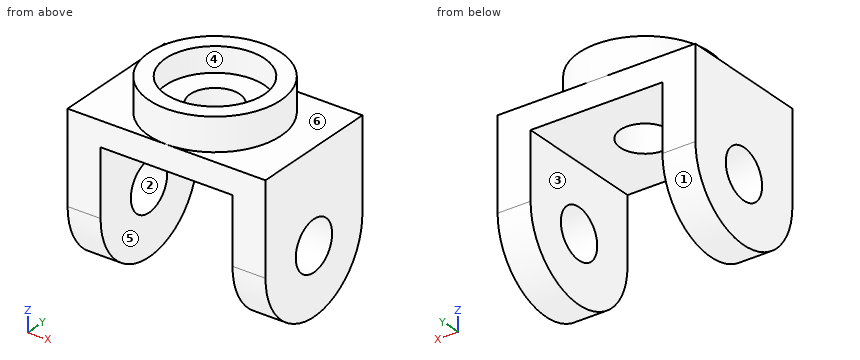
from build123d import *

# Parameters (mm, degrees)
SKETCH_W        = 120
SKETCH_H        = 80
PAD_DEPTH       = 15
SKETCH001_R     = 40
PAD001_DEPTH    = 20
SKETCH002_R     = 30
POCKET_DEPTH    = 15
SKETCH003_R     = 15
POCKET001_DEPTH = 20.001
SKETCH004_R     = 15
PAD002_DEPTH    = 120
SKETCH005_W     = 80
SKETCH005_H     = 96.232483
POCKET002_DEPTH = 80.0010000001


with BuildPart() as part:
    # Sketch → Pad (new body)
    with BuildSketch(Plane.XY):
        Rectangle(SKETCH_W, SKETCH_H)
    extrude(amount=-PAD_DEPTH)

    # Sketch001 → Pad001 (new body)
    with BuildSketch(Plane.XY):
        Circle(SKETCH001_R)
    extrude(amount=PAD001_DEPTH)

    # Sketch002 → Pocket (cut)
    with BuildSketch(Plane.XY.offset(20)):
        Circle(SKETCH002_R)
    extrude(amount=-POCKET_DEPTH, mode=Mode.SUBTRACT)

    # Sketch003 → Pocket001 (cut, through all)
    with BuildSketch(Plane.XY.offset(5)):
        Circle(SKETCH003_R)
    extrude(amount=-POCKET001_DEPTH, mode=Mode.SUBTRACT)

    # Sketch004 → Pad002 (new body)
    with BuildSketch(Plane.YZ.offset(60)):
        with BuildLine():
            ThreePointArc((-40, -55), (3.45478e-05, -95), (39.9999999999, -54.9999309045))
            Line((39.9999999999, -15), (39.9999999999, -54.9999309045))
            Line((-40, -15), (39.9999999999, -15))
            Line((-40, -55), (-40, -15))
        make_face()
        with Locations((0, -55)):
            Circle(SKETCH004_R, mode=Mode.SUBTRACT)
    extrude(amount=-PAD002_DEPTH)

    # Sketch005 → Pocket002 (cut, through all)
    with BuildSketch(Plane.XZ.offset(40)):
        with Locations((0, -63.1162415)):
            Rectangle(SKETCH005_W, SKETCH005_H)
    extrude(amount=-POCKET002_DEPTH, mode=Mode.SUBTRACT)


solid = part.part
Work out the finished part from the listing and answer in its coordinate system (mm). Face numbers are marked on the shaded views. A direction names the side the tool comes from. Round coordinates to 2 decimals unless told otherwise and drop trailing zeros. Loops run counter-clockwise (first coordinate to the right, second up) from the corner with the lowest first, then second, coordinate; pieces in that order, holes last. Notation, with made-up numbers: (-15, 52) - (30, 52) arc R24 ccw to (30, 75) - close; hole circle Ø11 at (24.5, -31.75). An arc over 180 degrees is marked (long way). One line per item, written item: value.
Q1. Each of these flat-tipped pins is pushed along its axis until it touches: pin 1 Ø5 at (x, y) = (14.5, 14) entering from +Z; pin 2 Ø1.5 at (x, z) = (-41.5, -68) entering from -Y; pin 3 Ø8 at (y, z) = (-3, -61.5) entering from +X; pin 4 Ø24 at (y, z) = (12, -59.5) entering from +X. Where does it stop, or does it pass through?
Check values:
pin 1: z = 5
pin 2: y = -38.08
pin 3: through
pin 4: x = 60
Q2. For the marked faces 4, 5 and 6, determine the directions among +Z, -Z, +X, -X, +Y, -Y from which every point of the face is accessible in a straight line to the end or side of a thin tool.
Check values:
face 4: +Z
face 5: -Z, +Y, -Y
face 6: +Z, +X
Q3. Find section B-B on y = 0. Give the vertices of the cut face in (x, z).
Check values:
outline: (-60, -95) - (-40, -95) - (-40, -70) - (-60, -70) - close; (-60, -40) - (-40, -40) - (-40, -15) - (-15, -15) - (-15, 5) - (-30, 5) - (-30, 20) - (-40, 20) - (-40, 0) - (-60, 0) - close; (15, -15) - (40, -15) - (40, -40) - (60, -40) - (60, 0) - (40, 0) - (40, 20) - (30, 20) - (30, 5) - (15, 5) - close; (40, -95) - (60, -95) - (60, -70) - (40, -70) - close
Q4. Find section A-A on z = -26. Give the vertices of the cut face in (x, y), and give its area (3 significant figures).
Check values:
outline: (-60, -40) - (-40, -40) - (-40, 40) - (-60, 40) - close; (40, -40) - (60, -40) - (60, 40) - (40, 40) - close
area: 3,200 mm2
Q5. Find section D-D on y = 32. Give the vertices of the cut face in (x, z), and give its area (3 significant figures).
Check values:
outline: (-60, -79) - (-40, -79) - (-40, -15) - (40, -15) - (40, -79) - (60, -79) - (60, 0) - (24, 0) - (24, 20) - (-24, 20) - (-24, 0) - (-60, 0) - close
area: 5,320 mm2
Q6. The mould has two halves that part along Z. Classify the marked faces 1, 2 and 3: +Z half, -Z half, draft (parallel to the pull), parting line (faces both ways), or undercut.
Check values:
face 1: -Z half
face 2: undercut
face 3: draft
Q7. Straight lines are drawn through the part: probe 1 along X at (y, z) = (30, -60.5); probe 2 along Y at (x, z) = (0, 10); probe 3 along Z at (x, y) = (33.5, 1). For each, find the intervals that lie inside material, in ascending order.
Check values:
probe 1: -60 to -40, 40 to 60
probe 2: -40 to -30, 30 to 40
probe 3: -15 to 20
Q8. Find section C-C on x = -9. Give the vertices of the cut face in (y, z), and give its area (3 significant figures).
Check values:
outline: (-40, -15) - (-12, -15) - (-12, 5) - (-28.62, 5) - (-28.62, 20) - (-38.97, 20) - (-38.97, 0) - (-40, 0) - close; (12, -15) - (40, -15) - (40, 0) - (38.97, 0) - (38.97, 20) - (28.62, 20) - (28.62, 5) - (12, 5) - close
area: 1,420 mm2
